```python
from build123d import *

# Parameters (mm, degrees)
SKETCH5_R          = 2.38125
CUT_EXTRUDE2_DEPTH = 10.664179163


with BuildPart() as part:
    # Sketch3 → Revolve1 (revolve)
    with BuildSketch(Plane(origin=(0, 0, 0), x_dir=(1, 0, 0), z_dir=(0, 1, 0))):
        Polygon((0, 0), (0, 38.1), (-9.525, 38.1), (-9.525, 28.575), (-3.314155064, 28.575), (-3.314155064, 15.875), (-9.664148049, 9.525007015), (-9.664148049, 7.015e-06), align=None)
    revolve(axis=Axis((-9.664148049, 0, -7.015e-06), (1, 0, 7.26e-07)))

    # Sketch5 → Cut-Extrude2 (cut, through all)
    with BuildSketch(Plane(origin=(-9.664151506, 0, -7.015e-06), x_dir=(-7.26e-07, 0, 1), z_dir=(-1, 0, -7.26e-07))):
        Circle(SKETCH5_R)
    extrude(amount=-CUT_EXTRUDE2_DEPTH, mode=Mode.SUBTRACT)


solid = part.part
```
CAD build for the part. Positions are in the model's coordinates, mm. A direction names the side the tool comes from. Give positions to 0.01 mm unless a question says otherwise; leave off trailing zeros. Order: outer loops, then holes, each group sorted by start corner. A loop starts at its lowest first (then second) coordinate and runs counter-clockwise, first axis right, second up. Notation, with made-up numbers: M 13.25,47.5 L 25.25,47.5 A27 ccw 25.25,84.5 Z; hole C 2,31 d5. An arc over 180 degrees is marked long. Put each result on its own line as item: value. Start each with the question number.
(1) Mould opens along Y. For faces 3 (the conical face through (-9.525, -28.347, 6.295)), 4 (the cylindrical face through (-4.829, -37.194, 8.259)), 5 (the conical face through (-9.356, 2.954, -9.379)), 6 (the cylindrical face through (-6.38, 28.33, 3.72)) say: +Y half, -Y half, draft (parallel to the pull), parting line (faces both ways), or undercut.
(2) Saw through at A-A, the plane y = 0. Write the cut outline in (x, z) (3 decimals), then the cut area to 3 significant figures.
(3) Flat gauge pins, fed straight in: pin 1 Ø2 at (x, z) = (-6.5, -16.5) entering from +Y; pin 2 Ø5 at (x, z) = (-6, -24.5) entering from -Y; pin 3 Ø5 at (x, z) = (-3.5, 2.5) entering from -Y. Where does each tip first touch, or does it go through?
(4) Saw through at B-B, the plane x = -6.25. Give the number of separate pieces and of enclosed holes in the cut face, then the cut area to 3 significant figures.
(5) Which spindle directions (+Z, -Z, +X, -X, +Y, -Y) get a long thin tool onto all of the face, cutting with end or side? Do faces 1 (the conical face through (-3.314, -16.099, 3.575)), 2 (the cylindrical face through (-4.9, -2.325, -0.516)). Say none if no direction does.
(6) Drill centre lines: line 1 along Y through (x, z) = (-5, -11); line 2 along Y through (x, z) = (-7.5, -7.5); line 3 along Y through (x, z) = (-4.75, -1). Where is each one in solid material? Low to high.
Check result:
1. face 3: draft
1. face 4: parting line
1. face 5: undercut
1. face 6: undercut
2. outline: M -9.664,-9.525 L -3.314,-15.875 L -3.314,-28.575 L -9.525,-28.575 L -9.525,-38.1 L 0,-38.1 L 0,-2.381 L -9.664,-2.381 Z; M -9.664,2.381 L 0,2.381 L 0,38.1 L -9.525,38.1 L -9.525,28.575 L -3.314,28.575 L -3.314,15.875 L -9.664,9.525 Z
2. area: 486 mm2
3. pin 1: stops at y = 34.8
3. pin 2: stops at y = -31.11
3. pin 3: stops at y = -38.1
4. separate pieces: 2
4. enclosed holes: 2
4. area: 2,500 mm2
5. face 1: -X
5. face 2: +X, -X
6. line 1: y = -36.48 to -26.37, -8.96 to 8.96, 26.37 to 36.48
6. line 2: y = -37.35 to -27.57, -8.97 to 8.97, 27.57 to 37.35
6. line 3: y = -38.09 to -28.56, -14.4 to -2.16, 2.16 to 14.4, 28.56 to 38.09
